CAD build for the part. Positions are in the model's coordinates, mm. Face numbers are marked on the shaded views. A direction names the side the tool comes from. Give positions to 0.01 mm unless a question says otherwise; leave off trailing zeros. Loops run counter-clockwise (first coordinate to the right, second up) from the corner with the lowest first, then second, coordinate; pieces in that order, holes last. Notation, with made-up numbers: M 49,50 L 82,50 A23 cw 82,65 Z; hole C 13.25,-25.75 d6. An arc over 180 degrees is marked long. One line per question, with ' | ' between items.
```python
from build123d import *

# Parameters (mm, degrees)
SKETCH1_R           = 6.5
BOSS_EXTRUDE1_DEPTH = 4
SKETCH2_R           = 5
BOSS_EXTRUDE2_DEPTH = 15
SKETCH3_R           = 1
BOSS_EXTRUDE3_DEPTH = 2
SKETCH4_W           = 1.1
SKETCH4_H           = 0.2


with BuildPart() as part:
    # Sketch1 → Boss-Extrude1 (new body)
    with BuildSketch(Plane(origin=(0, 0, 0), x_dir=(0, 0, -1), z_dir=(1, 0, 0))):
        Circle(SKETCH1_R)
    extrude(amount=BOSS_EXTRUDE1_DEPTH)

    # Sketch2 → Boss-Extrude2 (add)
    with BuildSketch(Plane.ZY):
        Circle(SKETCH2_R)
    extrude(amount=BOSS_EXTRUDE2_DEPTH)

    # Sketch3 → Boss-Extrude3 (add)
    with BuildSketch(Plane(origin=(4, 0, 0), x_dir=(0, 0, -1), z_dir=(1, 0, 0))):
        with Locations((0, 4)):
            Circle(SKETCH3_R)
    extrude(amount=BOSS_EXTRUDE3_DEPTH)

    # Sketch4 → Cut-Revolve1 (revolve, cut)
    with BuildSketch(Plane.XY):
        with Locations((-5.55, 4.9)):
            Rectangle(SKETCH4_W, SKETCH4_H)
    revolve(axis=Axis((-1.178470482, 0, 0), (-1, 0, 0)), mode=Mode.SUBTRACT)


solid = part.part
```
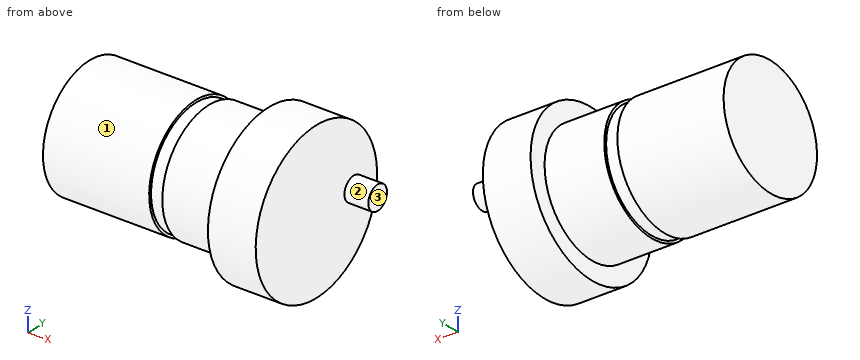
Item 1: Drop flat-ended pins along their axis: P1, Ø5, axis at x = 2, y = 5, coming from the -Z side; P2, Ø1.5, axis at x = -4, z = -4, coming from the -Y side; P3, Ø4, axis at y = 0, z = -5, coming from the +X side. Give the stop position or say it passes through.
Conclusion:
P1: z = -6 | P2: y = -3.8 | P3: x = 4
Item 2: Saw through at D-D on y = 1.75. Give the cut face in (x, z), and give its area (3 significant figures).
Conclusion:
outline: M -15,-4.68 L -6.1,-4.68 L -6.1,-4.47 L -5,-4.47 L -5,-4.68 L 0,-4.68 L 0,-6.26 L 4,-6.26 L 4,6.26 L 0,6.26 L 0,4.68 L -5,4.68 L -5,4.47 L -6.1,4.47 L -6.1,4.68 L -15,4.68 Z | area: 190 mm²
Item 3: Drill centre lines: line 1 along X through (y, z) = (0.75, 1.25); line 2 along X through (y, z) = (5.5, 0.5); line 3 along Y through (x, z) = (-1.75, 3.5). Where is each one in solid material? Low to high. Write a range as [from, to].
Conclusion:
line 1: [-15, 4] | line 2: [0, 4] | line 3: [-3.57, 3.57]
Item 4: 3-axis set-ups, long thin cutter, end or side, ignore diameter. For the marked faces 1, 2 and 3: which of +Z, -Z, +X, -X, +Y, -Y reach the whole face in a straight line?
Conclusion:
face 1: -X | face 2: +X | face 3: +Z, -Z, +X, +Y, -Y
Item 5: Saw through at B-B on z = 0. Give the cut face in (x, y).
Conclusion:
outline: M -15,-5 L -6.1,-5 L -6.1,-4.8 L -5,-4.8 L -5,-5 L 0,-5 L 0,-6.5 L 4,-6.5 L 4,3 L 6,3 L 6,5 L 4,5 L 4,6.5 L 0,6.5 L 0,5 L -5,5 L -5,4.8 L -6.1,4.8 L -6.1,5 L -15,5 Z
Item 6: Saw through at C-C on x = -12.5. Give the cut face in (y, z).
Conclusion:
outline: C 0,0 d10
Item 7: Saw through at A-A on y = 0. Give the cut face in (x, z).
Conclusion:
outline: M -15,-5 L -6.1,-5 L -6.1,-4.8 L -5,-4.8 L -5,-5 L 0,-5 L 0,-6.5 L 4,-6.5 L 4,6.5 L 0,6.5 L 0,5 L -5,5 L -5,4.8 L -6.1,4.8 L -6.1,5 L -15,5 Z
